The model under review builds one solid part; all positions refer to its coordinate system, in mm. Face numbers are marked on the shaded views. Give positions to 0.01 mm unless a question says otherwise; leave off trailing zeros. Write each loop counter-clockwise with the first axis right and the second up, starting at its lowest first coordinate (ties: lowest second). Pieces come first, ordered by that corner, then holes. Notation, with made-up numbers: (4, 70.25) - (33, 70.25) arc R24 ccw to (33, 107.25) - close; hole circle Ø5 at (49, 31). An arc over 180 degrees is marked (long way). Write item = value, one per line.
```python
from build123d import *

# Parameters (mm, degrees)
SKETCH_1_W          = 112
SKETCH_1_H          = 24
EXTRUDE_1_DEPTH     = 8
SKETCH_2_R          = 1.3
CUT_EXTRUDE_1_DEPTH = 30
SKETCH_3_R          = 2.5
SKETCH_3_R_2        = 1.5
CUT_EXTRUDE_2_DEPTH = 58.827329179
SKETCH_5_R          = 2.5
CUT_EXTRUDE_4_DEPTH = 1


with BuildPart() as part:
    # 草图1 → 凸台-拉伸1 (new body)
    with BuildSketch(Plane.XY):
        Rectangle(SKETCH_1_W, SKETCH_1_H)
    extrude(amount=EXTRUDE_1_DEPTH)

    # 草图2 → 切除-拉伸1 (cut)
    with BuildSketch(Plane(origin=(0, 12, 0), x_dir=(1, 0, 0), z_dir=(0, 1, 0))):
        with Locations(Location((-15, -4, 0), (0, 0, 270))):
            Circle(SKETCH_2_R)
        with Locations(Location((-45, -4, 0), (0, 0, 270))):
            Circle(SKETCH_2_R)
        with Locations(Location((45, -4, 0), (0, 0, 270))):
            Circle(SKETCH_2_R)
        with Locations(Location((15, -4, 0), (0, 0, 270))):
            Circle(SKETCH_2_R)
    extrude(amount=-CUT_EXTRUDE_1_DEPTH, mode=Mode.SUBTRACT)

    # 草图3 → 切除-拉伸2 (cut, through all)
    with BuildSketch(Plane(origin=(0, 0, 0), x_dir=(-1, 0, 0), z_dir=(0, 0, -1))):
        Circle(SKETCH_3_R)
        with Locations((-5.656854249, -5.656854249)):
            Circle(SKETCH_3_R_2)
        with Locations((-5.656854249, 5.656854249)):
            Circle(SKETCH_3_R_2)
        with Locations((5.656854249, 5.656854249)):
            Circle(SKETCH_3_R_2)
        with Locations((5.656854249, -5.656854249)):
            Circle(SKETCH_3_R_2)
    extrude(amount=-CUT_EXTRUDE_2_DEPTH, mode=Mode.SUBTRACT)

    # 草图5 → 切除-拉伸4 (cut)
    with BuildSketch(Plane.XY.offset(8)):
        with Locations((-5.656854249, -5.656854249)):
            Circle(SKETCH_5_R)
        with Locations((5.656854249, -5.656854249)):
            Circle(SKETCH_5_R)
        with Locations((5.656854249, 5.656854249)):
            Circle(SKETCH_5_R)
        with Locations((-5.656854249, 5.656854249)):
            Circle(SKETCH_5_R)
    extrude(amount=-CUT_EXTRUDE_4_DEPTH, mode=Mode.SUBTRACT)


solid = part.part
```
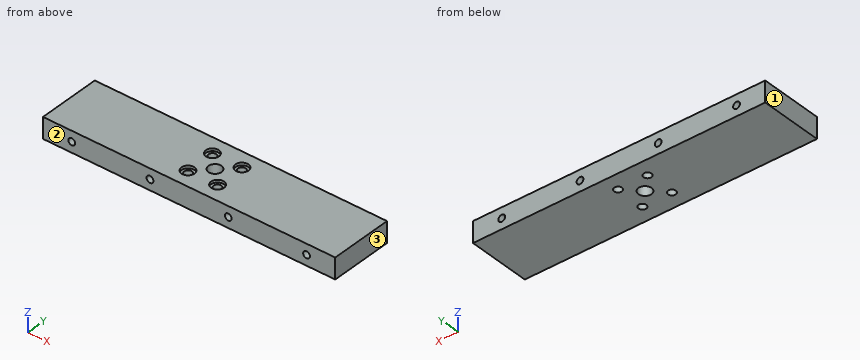
1. Insertion check: P1, Ø4, axis at x = 0, y = 0, coming from the +Z side; P2, Ø4, axis at x = 5.5, y = -5.5, coming from the +Z side. Each pin has a flat end and moves straight along its axis. Give the tip position at first contact, or say it passes through.
Findings below:
P1 = through
P2 = 7
2. For line 1 (X direction, y = 1.75, z = 4.25); line 2 (X direction, y = 0.5, z = 3.5); line 3 (X direction, y = -3.5, z = 3.25), list the stretches that pass through material, from the lowest coordinate up. Write a range as from..to.
Findings below:
line_1 = -56..-46.28, -43.72..-16.28, -13.72..-1.79, 1.79..13.72, 16.28..43.72, 46.28..56
line_2 = -56..-46.2, -43.8..-16.2, -13.8..-2.45, 2.45..13.8, 16.2..43.8, 46.2..56
line_3 = -56..-46.06, -43.94..-16.06, -13.94..13.94, 16.06..43.94, 46.06..56
3. Take a section at D-D on x = -45. Give the boundary of the cut face in (y, z), and give its area (3 significant figures).
Findings below:
outline = (-12, 0) - (12, 0) - (12, 2.7) - (-12, 2.7) - close; (-12, 5.3) - (12, 5.3) - (12, 8) - (-12, 8) - close
area = 130 mm²
4. Take a section at B-B on y = -9.25. Give the boundary of the cut face in (x, z), and give its area (3 significant figures).
Findings below:
outline = (-56, 0) - (56, 0) - (56, 8) - (-56, 8) - close; hole circle Ø2.6 at (-45, 4); hole circle Ø2.6 at (-15, 4); hole circle Ø2.6 at (15, 4); hole circle Ø2.6 at (45, 4)
area = 875 mm²
5. Take a section at C-C on x = 0. Give the boundary of the cut face in (y, z).
Findings below:
outline = (-12, 0) - (-2.5, 0) - (-2.5, 8) - (-12, 8) - close; (2.5, 0) - (12, 0) - (12, 8) - (2.5, 8) - close
6. Draft analysis for pull direction X (two halves, no side actions). For the marked faces 1, 2 and 3, state which applies: +X half, -X half, draft (parallel to the pull), parting line (faces both ways), or undercut.
Findings below:
face_1 = -X half
face_2 = draft
face_3 = +X half
7. Take a section at A-A on y = 0. Give the boundary of the cut face in (x, z), and give its area (3 significant figures).
Findings below:
outline = (-56, 0) - (-2.5, 0) - (-2.5, 8) - (-56, 8) - close; (2.5, 0) - (56, 0) - (56, 8) - (2.5, 8) - close; hole circle Ø2.6 at (-45, 4); hole circle Ø2.6 at (-15, 4); hole circle Ø2.6 at (15, 4); hole circle Ø2.6 at (45, 4)
area = 835 mm²
